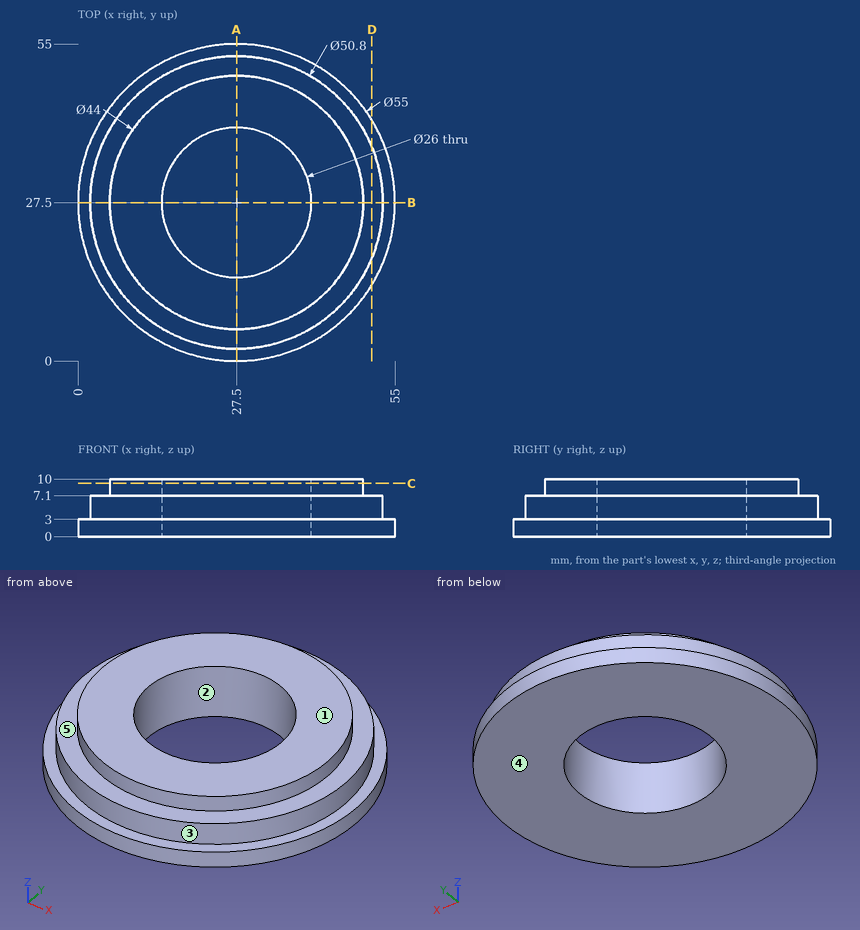
Part print with two shaded views. Sizes in mm from the minimum x, y, z corner. A direction names the side the tool comes from. Coordinates: 2 decimals unless noted, no trailing zeros. Write each loop counter-clockwise with the first axis right and the second up, starting at its lowest first coordinate (ties: lowest second). Pieces come first, ordered by that corner, then holes. Notation, with made-up numbers: (37.25, 78) - (67.25, 78) arc R10 cw to (67.25, 94) - close; hole circle Ø5 at (20.5, 71.25). An arc over 180 degrees is marked (long way). Put each result on its own line as item: value.
1. Flat gauge pins, fed straight in: pin 1 Ø5 at (x, z) = (26, 2.5) entering from -Y; pin 2 Ø5 at (x, y) = (47.5, 9) entering from -Z; pin 3 Ø6 at (x, z) = (24, 5) entering from +Y; pin 4 Ø1.5 at (y, z) = (19.5, 5) entering from -X. Where does each tip first touch, or does it go through?
Final values:
pin 1: stops at y = 0
pin 2: stops at z = 0
pin 3: stops at y = 54.97
pin 4: stops at x = 3.16
2. Band-saw the part on D-D (x = 51). Write the cut outline in (y, z).
Final values:
outline: (13.22, 0) - (41.78, 0) - (41.78, 3) - (37.14, 3) - (37.14, 7.1) - (17.86, 7.1) - (17.86, 3) - (13.22, 3) - close
3. 3-axis set-ups, long thin cutter, end or side, ignore diameter. For the marked faces 4 and 5: which of +Z, -Z, +X, -X, +Y, -Y reach the whole face in a straight line?
Final values:
face 4: -Z, +X, -X, +Y, -Y
face 5: +Z
4. Band-saw the part on C-C (z = 9.25). Write the cut outline in (x, y).
Final values:
outline: circle Ø44 at (27.5, 27.5); hole circle Ø26 at (27.5, 27.5)
5. Two-plate mould, pull along X, no slides. Class the marked faces 1, 2 and 3: +X half, -X half, draft (parallel to the pull), parting line (faces both ways), or undercut.
Final values:
face 1: draft
face 2: undercut
face 3: parting line
6. Probe line 1 along Y through (x, z) = (27.5, 4.5); line 2 along Y through (x, z) = (27.5, 7.75); line 3 along Z through (x, y) = (19.5, 3). List the from-to ranges inside material, lowest first. Write a range as [from, to].
Final values:
line 1: y = [2.1, 14.5], [40.5, 52.9]
line 2: y = [5.5, 14.5], [40.5, 49.5]
line 3: z = [0, 3]
7. Band-saw the part on A-A (x = 27.5). Write the cut outline in (y, z).
Final values:
outline: (0, 0) - (14.5, 0) - (14.5, 10) - (5.5, 10) - (5.5, 7.1) - (2.1, 7.1) - (2.1, 3) - (0, 3) - close; (40.5, 0) - (55, 0) - (55, 3) - (52.9, 3) - (52.9, 7.1) - (49.5, 7.1) - (49.5, 10) - (40.5, 10) - close
